Read the model definition and answer for the solid it produces. Units are mm, in the model's axes. Face numbers are marked on the shaded views. A direction names the side the tool comes from. Round coordinates to 2 decimals unless told otherwise and drop trailing zeros. Write each loop counter-clockwise with the first axis right and the second up, starting at its lowest first coordinate (ties: lowest second). Pieces come first, ordered by that corner, then holes. Notation, with made-up numbers: (41, 39) - (80, 39) arc R20 ccw to (80, 45) - close; hole circle Ø2 at (38.5, -3.5). An arc over 180 degrees is marked (long way). One line per item, written item: value. Start each with the question number.
(1) A cutting plane is placed at A-A, the plane z = -117. Determine the outline of the cut face in (x, y), plus the area to 3 significant figures.
(2) Find the intervals of material crossed by L1, parallel to Z at x = 44, y = -91.5; L2, parallel to Y at x = 0, z = 528; L3, parallel to Z at x = -9, y = 35.5, in increasing order.
(3) Flat-ended cylindrical pins translate along their axes: pin 1 Ø2 at (y, z) = (-56.5, 0.5) entering from +X; pin 2 Ø6 at (x, z) = (21.5, -644) entering from +Y; pin 3 Ø16 at (x, y) = (-58.21, 87.39) entering from +Z. Find the tip coordinate at first contact, or state that the pin passes through.
(4) A cutting plane is placed at B-B, the plane z = -725.5. Determine the outline of the cut face in (x, y), plus the area to 3 significant figures.
(5) For the marked faces 1 and 2, determine the directions among +Z, -Z, +X, -X, +Y, -Y from which every point of the face is accessible in a straight line to the end or side of a thin tool.
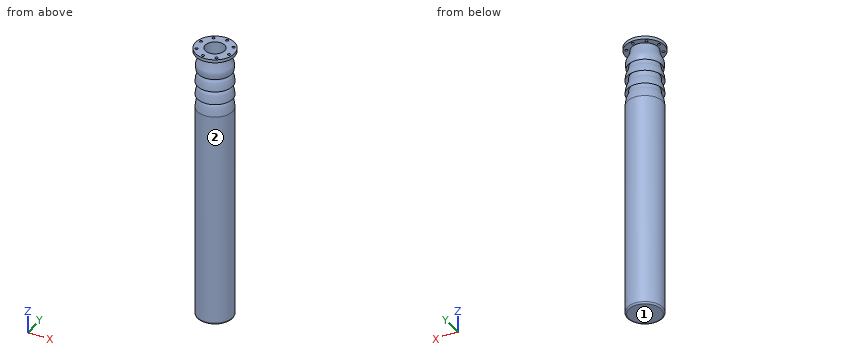
from build123d import *

# Parameters (mm, degrees)
F2_R            = 9
F3_DEPTH        = 20
F3_COPIES_COUNT = 8
F4_R            = 62.5
F5_DEPTH        = 1000
F6_R            = 10


# Not quite as in the source:
# - a pattern or mirror of a feature is missing from the dataset's text; its kind, count and spacing are read off the source's solid
# - a feature names something its author has since deleted; it is built from what else it names


with BuildPart() as f1:
    # F0 (on Front) → F1 (revolve)
    with BuildSketch(Plane.XZ):
        with BuildLine():
            Line((125, 796), (0, 796))
            Line((0, 796), (0, -989))
            Line((0, -989), (113.5784983635, -989))
            Line((113.5784983635, -989), (113.5784983635, 404.0072858334))
            add(Edge.make_bspline(
                [(92.1651435272, 507.9540014267), (92.9137259621, 470.1226269606), (100.84153647, 482.9142285433), (112.1166527424, 426.1022583198), (113.5784983635, 404.0072858334)],
                knots=[0, 0, 0, 0, 0.4424634244, 1, 1, 1, 1], degree=3))
            Line((92.1651435272, 507.9540014267), (113.5784983635, 487.6332684117))
            add(Edge.make_bspline(
                [(92.1651435272, 594.0558493723), (91.8360996428, 546.4974648718), (99.9002877175, 562.9049137477), (112.740117412, 507.2303715025), (113.5784983635, 487.6332684117)],
                knots=[0, 0, 0, 0, 0.4754834111, 1, 1, 1, 1], degree=3))
            Line((92.1651435272, 594.0558493723), (113.8892782108, 573.4401941299))
            add(Edge.make_bspline(
                [(92.1651435272, 666.1855578423), (92.9649518715, 631.6504081509), (100.208934103, 643.7752292593), (113.5784983635, 594.0558493723), (113.8892782108, 573.4401941299)],
                knots=[0, 0, 0, 0, 0.4429655486, 1, 1, 1, 1], degree=3))
            Line((92.1651435272, 666.1855578423), (107.2628746321, 651.8581922678))
            add(Edge.make_bspline(
                [(85, 776), (85.5159944694, 765.5527371234), (86.1594088799, 739.9492330129), (118.4720692878, 693.8768537198), (108.213278463, 662.5958632515), (107.2628746321, 651.8581922678)],
                knots=[0, 0, 0, 0, 0.3013801818, 0.6765769995, 1, 1, 1, 1], degree=3))
            Line((85, 776), (125, 776))
            Line((125, 776), (125, 796))
        make_face()
    revolve(axis=Axis((0, 0, -102), (0, 0, -1)))

    # F2 (on face) → F3 (cut, through all)
    with BuildSketch(Plane.XY.offset(796)):
        with Locations((20.6334079429, 102.9527196176)):
            Circle(F2_R)
    f3 = extrude(amount=-F3_DEPTH, mode=Mode.SUBTRACT)

    # F3_copies: F3 ×8 about axis
    f3_copies_axis = Axis((0, 0, 0), (0, 0, 1))
    for i in range(1, F3_COPIES_COUNT):
        add(f3.rotate(f3_copies_axis, i * 360 / F3_COPIES_COUNT), mode=Mode.SUBTRACT)

    # F4 (on face) → F5 (cut)
    with BuildSketch(Plane.XY.offset(796)):
        Circle(F4_R)
    extrude(amount=-F5_DEPTH, mode=Mode.SUBTRACT)

    # F6
    f6_edges = [f1.edges().sort_by_distance(p)[0] for p in [
        (-113.578498, 0, -989),
    ]]
    fillet(f6_edges, radius=F6_R)


solid = f1.part
Here are the results:
1. outline: circle Ø227.16 at (0, 0); hole circle Ø125 at (0, 0)
1. area: 28,300 mm²
2. L1: -989 to 465.8, 499.07 to 544, 585.17 to 628.66, 657.3 to 717.37, 776 to 796
2. L2: -106.98 to -62.5, 62.5 to 106.98
2. L3: -989 to -204
3. pin 1: x = 99.1
3. pin 2: y = 112.06
3. pin 3: z = 726.53
4. outline: circle Ø227.16 at (0, 0)
4. area: 40,500 mm²
5. face 1: -Z, +X, -X, +Y, -Y
5. face 2: -Z
